Geometry: final body of the model. Coordinates: model frame, mm. A direction names the side the tool comes from. Coordinates: 2 decimals unless noted, no trailing zeros. Write each loop counter-clockwise with the first axis right and the second up, starting at its lowest first coordinate (ties: lowest second). Pieces come first, ordered by that corner, then holes. Notation, with made-up numbers: (-13, 51) - (-9, 51) arc R13 cw to (-9, 61) - close; hole circle Ø2 at (-27, -23.75). An arc over 180 degrees is marked (long way). Put each result on its own line as item: value.
```python
from build123d import *

# Parameters (mm, degrees)
CUT_EXTRUDE1_DEPTH = 4
SKETCH3_W          = 6
SKETCH3_H          = 12.5


with BuildPart() as part:
    # Sketch1 → Revolve1 (revolve)
    with BuildSketch(Plane.XY, mode=Mode.PRIVATE) as revolve1_sk:
        with BuildLine():
            Line((0, -6), (0, -55))
            ThreePointArc((0, -55), (-1.464466094, -58.535533906), (-5, -60))
            Line((-5, -60), (-37, -60))
            ThreePointArc((-37, -60), (-40.535533906, -58.535533906), (-42, -55))
            Line((-42, -55), (-42, -45))
            ThreePointArc((-42, -45), (-40.535533906, -41.464466094), (-37, -40))
            Line((-37, -40), (-19, -40))
            ThreePointArc((-19, -40), (-15.464466094, -38.535533906), (-14, -35))
            Line((-14, -35), (-14, -6))
            Line((-14, -6), (0, -6))
        make_face()
    revolve(revolve1_sk.sketch.rotate(Axis((-33.627906977, 0, 0), (1, 0, 0)), 270), axis=Axis((-33.627906977, 0, 0), (1, 0, 0)))

    # Sketch2 → Cut-Extrude1 (cut)
    with BuildSketch(Plane.ZY.offset(14)):
        Polygon((4.948031545, -8.47645664), (9.814842556, 0.046892697), (4.866811012, 8.523349336), (-4.948031545, 8.47645664), (-9.814842556, -0.046892697), (-4.866811012, -8.523349336), align=None)
    extrude(amount=-CUT_EXTRUDE1_DEPTH, mode=Mode.SUBTRACT)

    # Sketch3 → Cut-Revolve1 (revolve, cut)
    with BuildSketch(Plane.XY, mode=Mode.PRIVATE) as cut_revolve1_sk:
        with Locations((-3, -6.25)):
            Rectangle(SKETCH3_W, SKETCH3_H)
    revolve(cut_revolve1_sk.sketch.rotate(Axis((-6, 0, 0), (1, 0, 0)), 270), axis=Axis((-6, 0, 0), (1, 0, 0)), mode=Mode.SUBTRACT)


solid = part.part
```
1. Section query C-C (x = -35). Return loops of the section in (y, z), then the cut area to 3 significant figures.
Answer below:
outline: circle Ø120 at (0, 0); hole circle Ø80 at (0, 0)
area: 6,280 mm²
2. Pin query (flat end, axial travel): pin 1 Ø8 at (x, z) = (-27, 46) entering from +Y; pin 2 Ø2 at (x, z) = (-32.5, -44) entering from +Y; pin 3 Ø19 at (y, z) = (-0.5, -4.5) entering from -X. Return the tip coordinate at first contact, or that it passes through.
Answer below:
pin 1: stops at y = 42.85
pin 2: stops at y = 41.84
pin 3: stops at x = -14
3. Section query A-A (x = -12.5). Return loops of the section in (y, z).
Answer below:
outline: circle Ø120 at (0, 0); hole (-8.52, -4.87) - (-0.05, -9.81) - (8.48, -4.95) - (8.52, 4.87) - (0.05, 9.81) - (-8.48, 4.95) - close
4. Ray query, probe 1 along Y at (x, z) = (-7.4, 0); probe 2 along X at (y, z) = (10.5, 30); probe 3 along Y at (x, z) = (-4, 0). Return the intervals inside material, ascending. Write a range as from..to.
Answer below:
probe 1: y = -60..-6, 6..60
probe 2: x = -14..0
probe 3: y = -59.9..-12.5, 12.5..59.9
5. Section query B-B (z = 0). Return loops of the section in (x, y), then the cut area to 3 significant figures.
Answer below:
outline: (-42, -55) arc R5 ccw to (-37, -60) - (-5, -60) arc R5 ccw to (0, -55) - (0, -12.5) - (-6, -12.5) - (-6, -6) - (-10, -6) - (-10, -8.5) - (-14, -8.5) - (-14, -35) arc R5 cw to (-19, -40) - (-37, -40) arc R5 ccw to (-42, -45) - close; (-42, 45) arc R5 ccw to (-37, 40) - (-19, 40) arc R5 cw to (-14, 35) - (-14, 8.5) - (-10, 8.5) - (-10, 6) - (-6, 6) - (-6, 12.5) - (0, 12.5) - (0, 55) arc R5 ccw to (-5, 60) - (-37, 60) arc R5 ccw to (-42, 55) - close
area: 2,510 mm²
6. Set-up query: faces 1 (the flat face through (-42, 40, -21)), 2 (the flat face through (-10, 6, 2)), 3 (the cylindrical face through (-2.958, -3.755, 11.923)). Return all of +Z, -Z, +X, -X, +Y, -Y with unobstructed straight access to the full face (end or side cutting, diameter ignored); none if empty.
Answer below:
face 1: +Z, -Z, -X, +Y, -Y
face 2: -X
face 3: +X
7. Mould query, pull axis Z, two halves, no side actions, for faces 4 (the flat face through (0, -13, 1)), 5 (the cylindrical face through (-21.22, -2.64, -59.94)), 6 (the cylindrical face through (-7.972, -1.802, 5.723)). Classes: +Z half, -Z half, draft (parallel to the pull), parting line (faces both ways), or undercut.
Answer below:
face 4: draft
face 5: parting line
face 6: undercut
